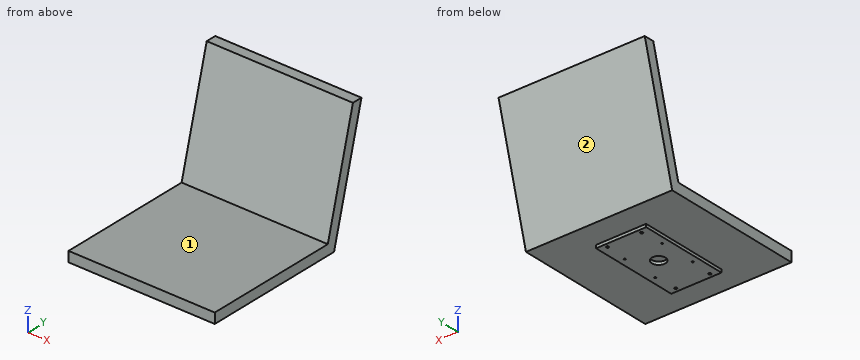
from build123d import *

# Parameters (mm, degrees)
F1_DEPTH      = 273.05
F1_DEPTH_BACK = 273.05
F2_R          = 4.7625
F2_R_2        = 3.175
F3_DEPTH      = 12.7
F4_W          = 187.325
F4_H          = 336.55
F4_R          = 4.7625
F4_R_2        = 3.175
F4_R_3        = 25.4
F5_DEPTH      = 11.1125


with BuildPart() as f1:
    # F0 (on Right) → F1 (new body, two sides)
    with BuildSketch(Plane.YZ) as f1_sk:
        Polygon((0, 38.1), (0, 0), (533.4, 0), (655.906371, 457.2), (617.806371, 457.2), (505.508864, 38.1), align=None)
    extrude(amount=F1_DEPTH)
    extrude(f1_sk.sketch, amount=-F1_DEPTH_BACK)

    # F2 (on face) → F3 (cut)
    with BuildSketch(Plane(origin=(0, 0, 0), x_dir=(1, 0, 0), z_dir=(0, 0, -1))):
        with Locations((-63.5, -114.3)):
            Circle(F2_R)
        with Locations((-63.5, -419.1)):
            Circle(F2_R)
        with Locations((63.5, -419.1)):
            Circle(F2_R)
        with Locations((69.85, -334.9625)):
            Circle(F2_R_2)
        with Locations((69.85, -198.4375)):
            Circle(F2_R_2)
        with Locations((-69.85, -198.4375)):
            Circle(F2_R_2)
        with Locations((-69.85, -334.9625)):
            Circle(F2_R_2)
        with Locations((63.5, -114.3)):
            Circle(F2_R)
    extrude(amount=-F3_DEPTH, mode=Mode.SUBTRACT)

    # F4 (on face) → F5 (join)
    with BuildSketch(Plane(origin=(0, 0, 0), x_dir=(1, 0, 0), z_dir=(0, 0, -1))):
        with Locations((0, -266.7)):
            Rectangle(F4_W, F4_H)
        with Locations((-63.5, -419.1)):
            Circle(F4_R, mode=Mode.SUBTRACT)
        with Locations((-69.85, -334.9625)):
            Circle(F4_R_2, mode=Mode.SUBTRACT)
        with Locations((63.5, -419.1)):
            Circle(F4_R, mode=Mode.SUBTRACT)
        with Locations((69.85, -334.9625)):
            Circle(F4_R_2, mode=Mode.SUBTRACT)
        with Locations((-69.85, -198.4375)):
            Circle(F4_R_2, mode=Mode.SUBTRACT)
        with Locations((-63.5, -114.3)):
            Circle(F4_R, mode=Mode.SUBTRACT)
        with Locations((0, -266.7)):
            Circle(F4_R_3, mode=Mode.SUBTRACT)
        with Locations((69.85, -198.4375)):
            Circle(F4_R_2, mode=Mode.SUBTRACT)
        with Locations((63.5, -114.3)):
            Circle(F4_R, mode=Mode.SUBTRACT)
    extrude(amount=F5_DEPTH)


solid = f1.part
Work out the finished part from the listing and answer in its coordinate system (mm). Face numbers are marked on the shaded views. A direction names the side the tool comes from. Round coordinates to 2 decimals unless told otherwise and drop trailing zeros. Write each loop counter-clockwise with the first axis right and the second up, starting at its lowest first coordinate (ties: lowest second). Pieces come first, ordered by that corner, then holes. Notation, with made-up numbers: (18, 48.5) -> (50, 48.5) arc R29 cw to (50, 83.5) -> close; hole circle Ø5 at (89, 21.25). An arc over 180 degrees is marked (long way). Answer as CSV lines item,"result". Start each with the question number.
(1) A tool of negligible diameter and unlimited length cuts with its end or side. For the marked faces 1 and 2, from which of +Z, -Z, +X, -X, +Y, -Y can it reach the whole face along a straight path? Write none if from no direction.
(2) Find the intervals of material crossed by probe 1 along Y at (x, z) = (-63.5, -2.75) (1 decimal); probe 2 along X at (y, z) = (419, -1); probe 3 along Y at (x, z) = (-69.85, -5) (1 decimal), in increasing order.
(3) The part is cut by section A-A, the plane y = 386.5. Give the vertices of the cut face in (x, z), then the cut area to 3 significant figures.
(4) Each of these flat-tipped pins is pushed along its axis until it touches: pin 1 (1 mm diameter, centred on x = 209.5, y = 208, fed in from +Z); pin 2 (8.5 mm diameter, centred on x = -63.5, y = 114.3, fed in from -Z); pin 3 (12 mm diameter, centred on x = -4, z = -7, fed in from -Y) (3 decimals); pin 4 (12 mm diameter, centred on y = 209.5, z = -3.5, fed in from -X). Where does it stop, or does it pass through?
(5) The part is cut by section D-D, the plane x = -133. Give the vertices of the cut face in (y, z), then the cut area to 3 significant figures.
(6) The part is cut by section C-C, the plane y = 266.7. Give the vertices of the cut face in (x, z), then the cut area to 3 significant figures.
(7) The part is cut by section B-B, the plane x = 39. Give the vertices of the cut face in (y, z) (1 decimal), then the cut area to 3 significant figures.
Output values:
1,face 1,"+Z, +X, -X, -Y"
1,face 2,"-Z, +X, -X, +Y"
2,probe 1,"y = 98.4 to 109.5, 119.1 to 414.3, 423.9 to 435"
2,probe 2,"x = -93.66 to -68.26, -58.74 to 58.74, 68.26 to 93.66"
2,probe 3,"y = 98.4 to 195.3, 201.6 to 331.8, 338.1 to 435"
3,outline,"(-273.05, 0) -> (-93.66, 0) -> (-93.66, -11.11) -> (93.66, -11.11) -> (93.66, 0) -> (273.05, 0) -> (273.05, 38.1) -> (-273.05, 38.1) -> close"
3,area,"22,900 mm²"
4,pin 1,"stops at z = 38.1"
4,pin 2,"stops at z = 12.7"
4,pin 3,"stops at y = 98.425"
4,pin 4,"stops at x = -273.05"
5,outline,"(0, 0) -> (533.4, 0) -> (655.91, 457.2) -> (617.81, 457.2) -> (505.51, 38.1) -> (0, 38.1) -> close"
5,area,"36,500 mm²"
6,outline,"(-273.05, 0) -> (-93.66, 0) -> (-93.66, -11.11) -> (-25.4, -11.11) -> (-25.4, 0) -> (25.4, 0) -> (25.4, -11.11) -> (93.66, -11.11) -> (93.66, 0) -> (273.05, 0) -> (273.05, 38.1) -> (-273.05, 38.1) -> close"
6,area,"22,300 mm²"
7,outline,"(0, 0) -> (98.4, 0) -> (98.4, -11.1) -> (435, -11.1) -> (435, 0) -> (533.4, 0) -> (655.9, 457.2) -> (617.8, 457.2) -> (505.5, 38.1) -> (0, 38.1) -> close"
7,area,"40,200 mm²"
